```python
from build123d import *

# Parameters (mm, degrees)
SKETCH1_R               = 30
SKETCH1_R_2             = 20
BOSS_EXTRUDE1_DEPTH     = 10
CUT_EXTRUDE1_DEPTH      = 44.588989435
CUT_EXTRUDE1_DEPTH_BACK = 44.588989435
SKETCH2_R               = 3
SCALE1_SCALE            = 0.35


with BuildPart() as part:
    # Sketch1 → Boss-Extrude1 (new body)
    with BuildSketch(Plane.XY):
        Circle(SKETCH1_R)
        Circle(SKETCH1_R_2, mode=Mode.SUBTRACT)
    extrude(amount=BOSS_EXTRUDE1_DEPTH)

    # Sketch2 → Cut-Extrude1 (cut, two sides: drawn at the far end of the back side and taken through both)
    with BuildSketch(Plane(origin=(0, 0, 0), x_dir=(1, 0, 0), z_dir=(0, 1, 0)).offset(-CUT_EXTRUDE1_DEPTH_BACK)):
        with Locations(Location((0, -5, 0), (0, 0, 270))):
            Circle(SKETCH2_R)
    extrude(amount=CUT_EXTRUDE1_DEPTH + CUT_EXTRUDE1_DEPTH_BACK, mode=Mode.SUBTRACT)


with BuildPart() as part_1:
    # Scale1: scaled about (-0.001116422, 0, 4.999941886)
    add(part.part.scale(SCALE1_SCALE).moved(Location((-0.000725674, 0, 3.249962226))))


solid = part_1.part
```
Part model, mm, in its own coordinate system. Round coordinates to 2 decimals unless told otherwise and drop trailing zeros. Loops run counter-clockwise (first coordinate to the right, second up) from the corner with the lowest first, then second, coordinate; pieces in that order, holes last.
Item 1: Cut at B-B, the plane x = -3.5. Give the cut face in (y, z), then the cut area to 3 significant figures.
Item 2: Cut at C-C, the plane x = -8. Give the cut face in (y, z).
Item 3: Drill centre lines: line 1 (Y direction, x = 1, z = 6.1); line 2 (Y direction, x = -5, z = 4.6); line 3 (X direction, y = 2, z = 4.7). Where is each one in solid material? Low to high.
Item 4: Drop a flat-ended pin along its axis: P1, Ø1.5, axis at x = -1, z = 5, coming from the -Y side. Give the stop position or say it passes through.
Item 5: Mould opens along X. For faces 1 (the face through (10, 3.2, 5)), 2 (the face through (0.315, 8.684, 6.001)), 3 (the face through (2, -7, 3.25)) say: +X half, -X half, draft (parallel to the pull), parting line (faces both ways), or undercut.
Item 6: Cut at A-A, the plane y = 0. Give the cut face in (x, z), then the cut area to 3 significant figures.
A:
1. outline: (-9.9, 3.25) - (-6.06, 3.25) - (-6.06, 6.75) - (-9.9, 6.75) - close; (6.06, 3.25) - (9.9, 3.25) - (9.9, 6.75) - (6.06, 6.75) - close
1. area: 26.9 mm2
2. outline: (-6.8, 3.25) - (6.8, 3.25) - (6.8, 6.75) - (-6.8, 6.75) - close
3. line 1: y = -10.45 to -6.93, 6.93 to 10.45
3. line 2: y = -9.23 to -4.9, 4.9 to 9.23
3. line 3: x = -10.31 to -6.71, 6.71 to 10.31
4. P1: stops at y = -10.47
5. face 1: parting line
5. face 2: undercut
5. face 3: draft
6. outline: (-10.5, 3.25) - (-7, 3.25) - (-7, 6.75) - (-10.5, 6.75) - close; (7, 3.25) - (10.5, 3.25) - (10.5, 6.75) - (7, 6.75) - close
6. area: 24.5 mm2
